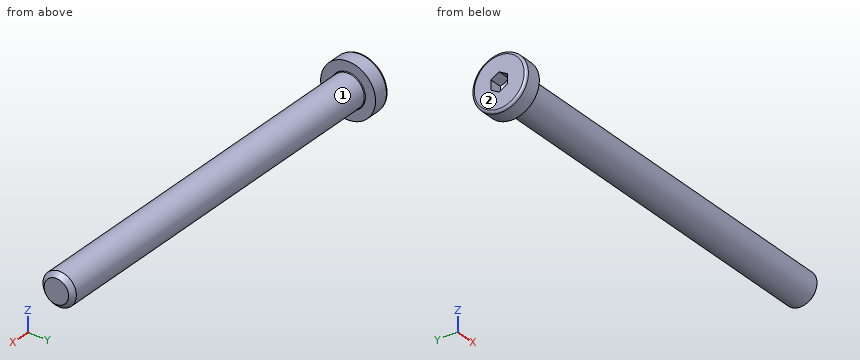
Autodesk Inventor part; units mm, degrees
ref_plane "Work Plane1" through (29, 0, 0) normal (0, -1, 0) x (1, 0, 0)
ref_plane "YZ Plane" through (0, 0, 0) normal (1, 0, 0) x (0, 1, 0)
ref_plane "XZ Plane" through (0, 0, 0) normal (0, 1, 0) x (-1, 0, 0)
sketch "Sketch1" plane through (0, 0, 0) normal (0, 0, 1) x (1, 0, 0)
  line L0 (0.1334, 0) -> (57.15, 0)
  line L1 (57.15, 0) -> (57.15, 2.413)
  line L2 (57.15, 2.413) -> (34.925, 2.413)
  line L3 (34.925, 2.413) -> (32.8082, 2.413)
  line L4 (32.8082, 2.413) -> (0, 2.413)
  line L5 (0, 2.413) -> (0, 3.9624)
  line L6 (0, 3.9624) -> (-2.4892, 3.9624)
  line L7 (-2.4892, 3.9624) -> (-2.4892, 1.3748)
  line L8 (-2.4892, 1.3748) -> (-0.6604, 1.3748)
  line L9 (-0.6604, 1.3748) -> (0.1334, 0)
  line L10 (-14.417, 0) -> (69.0778, 0)
  line L11 (0, -0.7925) -> (0, 4.7549)
  line L12 (34.925, 2.413) -> (0, 2.413) construction
  dimension "d1" = 22.225
  dimension "d2" = 2.1168
  dimension "d3" = 2.4892
  dimension "d4" = 1.8288
  dimension "d5" = 60
  dimension "d6" = 4.826
  dimension "d7" = 4.826
  dimension "d8" = 2.7496
  dimension "d9" = 7.9248
  dimension "d26" = 57.15
revolve "Body" add sketch "Sketch1" angle 360 about axis through (0.1334, 0, 0) along (1, 0, 0) contours L9 L11 L4 L3 L2 L1 L0 | L9 L8 L7 L6 L5 L11
sketch "Sketch2" plane through (-2.4892, 0, 0) normal (-1, 0, 0) x (0, 0, 1)
  circle A0 centre (0, 0) radius 1.3748
  line L0 (0, -5.5474) -> (0, 5.5474)
  line L1 (-5.5474, 0) -> (5.5474, 0)
  line L2 (1.3748, 0) -> (0.6874, -1.1906)
  line L3 (0.6874, -1.1906) -> (-0.6874, -1.1906)
  line L4 (-0.6874, -1.1906) -> (-1.3748, 0)
  line L5 (-1.3748, 0) -> (-0.6874, 1.1906)
  line L6 (-0.6874, 1.1906) -> (0.6874, 1.1906)
  line L7 (0.6874, 1.1906) -> (1.3748, 0)
extrude "Slot" add sketch "Sketch2" against normal up to next contours L7 A0 | A0 L2 | L6 L0 A0 | A0 L0 L3 | L0 L6 A0 | A0 L3 L0 | L4 A0 | A0 L5
fillet "Fillet1" radius 0.3556 1 edges at (-2.4892, -3.9624, 0)
thread "Thread"
chamfer "Chamfer1" distance 0.6492 distance2 0.6492 1 edges at (57.15, -2.413, 0) measured on face at (57.15, -0.4231, -0.1925)
ref_plane "Work Plane1" through (29, 0, 0) normal (0, -1, 0) x (1, 0, 0)
fillet "Fillet2" radius 0.1 1 edges at (0, -2.413, 0)
equation "\"d1\" = GEL"
equation "\"d3\" = KOH"
equation "\"d4\" = INTI"
equation "\"d6\" = GD"
equation "\"d7\" = BDM"
equation "\"d8\" = 1.1547 * SW"
equation "\"d9\" = KOD"
equation "\"d26\" = NLG"
equation "\"d30\" = R"
equation "\"d17\" = RR"
equation "\"d13\" = GEL"
equation "\"d15\" = -0.5 * SPD + 0.5 * GD"
equation "\"d16\" = GUL"
equation "\"GD\" = NND"
equation "\"NLG\" = 57.15"
equation "\"GEL\" = 22.225"
equation "\"KOD\" = 7.9248"
equation "\"KOH\" = 2.4892"
equation "\"INTI\" = 1.8288"
equation "\"GAL\" = 2.11668"
equation "\"GUL\" = 0.64922"
equation "\"BDM\" = NND"
equation "\"SW\" = 2.38125"
equation "\"RR\" = 0.3556"
equation "\"SPD\" = GD1"
equation "\"R\" = 0.1"
equation "\"PHH\" = 0.24892"
equation "\"THREADDIA\" = 4.826"
equation "\"FAWI\" = 45deg"
equation "\"NND\" = 4.826"
equation "\"E0\" = 1.155 * SW"
equation "\"FAWI1\" = 30deg"
equation "\"TOA\" = 30deg"
equation "\"GD1\" = 3.52755"
properties part number "Unbrako - 10 x 2 1/4" material "Steel, Mild"
Model file for the job. Use its own axes, mm. Face numbers are marked on the shaded views. A direction names the side the tool comes from. Coordinates: 2 decimals unless noted, no trailing zeros. Order: outer loops, then holes, each group sorted by start corner. A loop starts at its lowest first (then second) coordinate and runs counter-clockwise, first axis right, second up. Notation, with made-up numbers: (19.25, 1) - (65.25, 1) arc R26 cw to (65.25, 38) - close; hole circle Ø9 at (-9.75, -1.5). An arc over 180 degrees is marked (long way). Return JSON: item names as keys, results as strings. Group by question number.
1) Probe line 1 (X direction, y = -0.75, z = -3); line 2 (Y direction, x = 26.5, z = 2); line 3 (Y direction, x = 22, z = -0.75). List the from-to ranges inside material, lowest first. Write a range as from..to.
2) Flat gauge pins, fed straight in: P1, Ø2, axis at x = 43.5, z = -0.5, coming from the -Y side; P2, Ø1.5, axis at x = -1, z = 0.5, coming from the -Y side; P3, Ø1.5, axis at x = 26.5, y = -1, coming from the -Z side; P4, Ø2, axis at x = 48, y = -1, coming from the +Z side. Where does each tip first touch, or does it go through?
3) Saw through at A-A, the plane x = 43. Write the cut outline in (y, z), plus the area to 3 significant figures.
4) Tool access for the marked faces 1 and 2: list every direction of +Z, -Z, +X, -X, +Y, -Y with a clear straight run to the whole face (end or side of a thin tool).
Values found:
{
 "1": {"line 1": "x = -2.49..0", "line 2": "y = -1.35..1.35", "line 3": "y = -2.29..2.29"},
 "2": {"P1": "stops at y = -2.41", "P2": "stops at y = -3.96", "P3": "stops at z = -2.4", "P4": "stops at z = 2.41"},
 "3": {"outline": "circle Ø4.83 at (0, 0)", "area": "18.3 mm²"},
 "4": {"face 1": "+X", "face 2": "+Z, -Z, -X, +Y, -Y"}
}
